Geometry check sheet. Reference: the model listing, model coordinates, mm. Coordinates: 2 decimals unless noted, no trailing zeros. Write each loop counter-clockwise with the first axis right and the second up, starting at its lowest first coordinate (ties: lowest second). Pieces come first, ordered by that corner, then holes. Notation, with made-up numbers: (45.25, 62.25) -> (84.25, 62.25) arc R19 cw to (84.25, 66.25) -> close; hole circle Ø11 at (26, 47.25). An arc over 180 degrees is marked (long way). Answer in a Markdown table with one row per item. Add a question column.
Q1. Release check for a two-part mould opening along Y. For faces 1 (the face through (3.802, -6.465, 4.437)), 2 (the face through (3.698, 6.526, 4.437)), 3 (the face through (2.046, 3.935, 4.437)), 4 (the face through (3, -4, 0)) record: pulls with the +Y half, pulls with the -Y half, needs draft (parallel to the pull), parting line crosses it, or undercut.
Q2. Section check B-B, the plane x = -1. Record the boundary of the cut face in (y, z), and give its area (3 significant figures).
Q3. Section check D-D, the plane y = 6.25. Record the boundary of the cut face in (x, z), and give its area (3 significant figures).
Q4. Section check A-A, the plane y = 0. Record the boundary of the cut face in (x, z) (3 decimals).
Q5. Gauge pin test, flat end, axial feed: P1, Ø4, axis at x = 4, z = 7.5, coming from the +Y side. Record the tip position at first contact, or that the pin passes through.
Q6. Thickness scan on line 1 (X direction, y = -0.5, z = 6.75); line 2 (X direction, y = -1.75, z = 1.75); line 3 (Y direction, x = 3.5, z = 7.5). Record the ranges inside material, lowest first.
Q7. Section check C-C, the plane z = 0.5. Record the boundary of the cut face in (x, y) (3 decimals).
Autodesk Inventor part; units mm, degrees
ref_plane "YZ Plane" through (0, 0, 0) normal (1, 0, 0) x (0, 1, 0)
ref_plane "XZ Plane" through (0, 0, 0) normal (0, 1, 0) x (-1, 0, 0)
ref_plane "XY Plane" through (0, 0, 0) normal (0, 0, 1) x (1, 0, 0)
sketch "Sketch1" plane through (0, 0, 0) normal (0, 0, 1) x (1, 0, 0)
  circle A0 centre (0, 0) radius 4.435
  line L0 (0, 8.6603) -> (7.5, 4.3301)
  line L1 (7.5, 4.3301) -> (7.5, -4.3301)
  line L2 (7.5, -4.3301) -> (0, -8.6603)
  line L3 (0, -8.6603) -> (-7.5, -4.3301)
  line L4 (-7.5, -4.3301) -> (-7.5, 4.3301)
  line L5 (-7.5, 4.3301) -> (0, 8.6603)
  dimension "d0" = 8.87
  dimension "d3" = 15
extrude "Extrusion1" add sketch "Sketch1" along normal blind 9
thread "Thread1"
properties part number "EEThreadedRodNut"
Calculated:
| question | item | result |
|---|---|---|
| 1 | face 1 | pulls with the -Y half |
| 1 | face 2 | pulls with the +Y half |
| 1 | face 3 | undercut |
| 1 | face 4 | needs draft |
| 2 | outline | (-8.08, 0) -> (-4.32, 0) -> (-4.32, 9) -> (-8.08, 9) -> close; (4.32, 0) -> (8.08, 0) -> (8.08, 9) -> (4.32, 9) -> close |
| 2 | area | 67.7 mm² |
| 3 | outline | (-4.17, 0) -> (4.17, 0) -> (4.17, 9) -> (-4.17, 9) -> close |
| 3 | area | 75.1 mm² |
| 4 | outline | (-7.5, 0) -> (-4.435, 0) -> (-4.435, 9) -> (-7.5, 9) -> close; (4.435, 0) -> (7.5, 0) -> (7.5, 9) -> (4.435, 9) -> close |
| 5 | P1 | stops at y = 7.51 |
| 6 | line 1 | x = -7.5 to -4.41, 4.41 to 7.5 |
| 6 | line 2 | x = -7.5 to -4.08, 4.08 to 7.5 |
| 6 | line 3 | y = -6.64 to -2.72, 2.72 to 6.64 |
| 7 | outline | (-7.5, -4.33) -> (0, -8.66) -> (7.5, -4.33) -> (7.5, 4.33) -> (0, 8.66) -> (-7.5, 4.33) -> close; hole circle Ø8.87 at (0, 0) |
